from build123d import *

# Parameters (mm, degrees)
SKETCH1_R           = 18
SKETCH1_R_2         = 3
SKETCH1_R_3         = 3.628209061
BOSS_EXTRUDE1_DEPTH = 16.65
SKETCH2_W           = 30
SKETCH2_H           = 12.65
CUT_EXTRUDE2_DEPTH  = 11
CUT_EXTRUDE3_REACH  = 171.197
SKETCH3_R           = 4.5
FILLET2_R           = 1


with BuildPart() as part:
    # Sketch1 → Boss-Extrude1 (new body)
    with BuildSketch(Plane(origin=(0, 0, 0), x_dir=(1, 0, 0), z_dir=(0, 1, 0))):
        with BuildLine():
            Line((-1.087094723, -18.968875166), (-157.872155118, -9.983618508))
            ThreePointArc((-157.872155118, -9.983618508), (-167.3, 0), (-157.872155118, 9.983618508))
            Line((-157.872155118, 9.983618508), (-1.087094723, 18.968875166))
            ThreePointArc((-1.087094723, 18.968875166), (0, 19), (1.087094723, 18.968875166))
            Line((1.087094723, 18.968875166), (157.872155118, 9.983618508))
            ThreePointArc((157.872155118, 9.983618508), (167.3, 0), (157.872155118, -9.983618508))
            Line((157.872155118, -9.983618508), (1.087094723, -18.968875166))
            ThreePointArc((1.087094723, -18.968875166), (0, -19), (-1.087094723, -18.968875166))
        make_face()
        Circle(SKETCH1_R, mode=Mode.SUBTRACT)
        with Locations(Location((-157.3, 0, 0), (0, 0, 270))):
            Circle(SKETCH1_R_2, mode=Mode.SUBTRACT)
        with Locations(Location((157.3, 0, 0), (0, 0, 270))):
            Circle(SKETCH1_R_3, mode=Mode.SUBTRACT)
        Circle(SKETCH1_R)
    extrude(amount=BOSS_EXTRUDE1_DEPTH)

    # Sketch2 → Cut-Extrude2 (cut, symmetric)
    with BuildSketch(Plane(origin=(-157.3, 0, 0), x_dir=(0, 0, -1), z_dir=(1, 0, 0))):
        with Locations((0, 8.325)):
            Rectangle(SKETCH2_W, SKETCH2_H)
    cut_extrude2 = extrude(amount=CUT_EXTRUDE2_DEPTH, both=True, mode=Mode.SUBTRACT)

    # Mirror1: Cut-Extrude2 across plane
    add(cut_extrude2.mirror(Plane(origin=(0, 0, 0), x_dir=(0, 0, 1), z_dir=(1, 0, 0))), mode=Mode.SUBTRACT)

    # Sketch3 → Cut-Extrude3 (cut, up to next)
    with BuildSketch(Plane(origin=(0, 16.65, 0), x_dir=(1, 0, 0), z_dir=(0, 1, 0)), mode=Mode.PRIVATE) as cut_extrude3_sk1:
        with Locations(Location((0, 0, 0), (0, 0, 270))):
            Circle(SKETCH3_R)
    cut_extrude3_tool1 = extrude(cut_extrude3_sk1.sketch, amount=-CUT_EXTRUDE3_REACH, mode=Mode.PRIVATE) & part.part
    add(cut_extrude3_tool1.solids().sort_by_distance((0, 16.65, 0))[0], mode=Mode.SUBTRACT)

    # Fillet2
    fillet2_edges = [part.edges().sort_by_distance(p)[0] for p in [
        (-167.3, 2, 0),
        (-167.3, 14.65, 0),
        (-152.086077559, 14.65, 10.315215102),
        (-152.086077559, 2, 10.315215102),
        (-152.086077559, 14.65, -10.315215102),
        (-152.086077559, 2, -10.315215102),
        (152.086077559, 2, -10.315215102),
        (167.3, 2, 0),
        (167.3, 14.65, 0),
        (152.086077559, 14.65, -10.315215102),
        (152.086077559, 2, 10.315215102),
        (152.086077559, 14.65, 10.315215102),
    ]]
    fillet(fillet2_edges, radius=FILLET2_R)


solid = part.part
Verification items for the finished model (mm, model axes). A direction names the side the tool comes from. Coordinates: 2 decimals unless noted, no trailing zeros. Write each loop counter-clockwise with the first axis right and the second up, starting at its lowest first coordinate (ties: lowest second). Pieces come first, ordered by that corner, then holes. Notation, with made-up numbers: (55.25, 19.25) - (72.25, 19.25) arc R20 cw to (72.25, 29.25) - close; hole circle Ø5 at (9.25, 19). An arc over 180 degrees is marked (long way). Answer as a JSON object with one key per item and string values.
(1) Cross-section at A-A on y = 4.5. Record the cut outline in (x, z).
Report:
{"outline": "(-146.3, -10.65) - (-1.09, -18.97) arc R19 ccw to (1.09, -18.97) - (146.3, -10.65) - (146.3, 10.65) - (1.09, 18.97) arc R19 ccw to (-1.09, 18.97) - (-146.3, 10.65) - close; hole circle Ø9 at (0, 0)"}
(2) Mould release check, pull along Z, two halves, no side actions. Record for faces 1 (the cylindrical face through (1.352, 8.442, 4.292)), 2 (the flat face through (78.38, 8.21, -14.54)), 3 (the flat face through (154, 14.65, 2)), 4 (the cylindrical face through (-167.3, 0.5, 0.2)): pulls with the +Z half, pulls with the -Z half, needs draft (parallel to the pull), parting line crosses it, or undercut.
Report:
{"face 1": "undercut", "face 2": "pulls with the -Z half", "face 3": "needs draft", "face 4": "parting line crosses it"}
(3) Thickness scan on line 1 along X through (y, z) = (0.7, 0); line 2 along Z through (x, y) = (-0.5, 6.5); line 3 along Z through (x, y) = (157.3, 1.25). Record the ranges inside material, lowest first.
Report:
{"line 1": "-167.3 to -160.3, -154.3 to -4.5, 4.5 to 153.67, 160.93 to 167.3", "line 2": "-18.99 to -4.47, 4.47 to 18.99", "line 3": "-9.98 to -3.63, 3.63 to 9.98"}
(4) Tool access check on faces 5 (the flat face through (154, 2, 2)), 6 (the cylindrical face through (160.897, 0.986, -0.472)). Record the directions out of +Z, -Z, +X, -X, +Y, -Y that give a thin tool (end or side, any length) a straight path to the whole face; none if there is none.
Report:
{"face 5": "+Z, -Z, +X", "face 6": "+Y, -Y"}
(5) Cross-section at C-C on x = 53.5. Record the cut outline in (y, z).
Report:
{"outline": "(0, -15.97) - (16.65, -15.97) - (16.65, 15.97) - (0, 15.97) - close"}
(6) Cross-section at D-D on x = -35. Record the cut outline in (y, z).
Report:
{"outline": "(0, -17.03) - (16.65, -17.03) - (16.65, 17.03) - (0, 17.03) - close"}
(7) Gauge pin test, flat ends, axial feed: pin 1 Ø8 at (x, y) = (-48.5, 13) entering from +Z; pin 2 Ø3 at (y, z) = (3, -2.5) entering from -X; pin 3 Ø4.5 at (y, z) = (5, 0) entering from -X. Record the tip position at first contact, or that the pin passes through.
Report:
{"pin 1": "z = 16.48", "pin 2": "x = -166.91", "pin 3": "x = -146.3"}
(8) Cross-section at B-B on z = 0. Give the number of separate pieces and of enclosed holes in the cut face, plus the area to 3 significant figures.
Report:
{"separate pieces": "6", "enclosed holes": "0", "area": "4,840 mm^2"}
